Autodesk Inventor part; units mm, degrees
ref_plane "YZ Plane" through (0, 0, 0) normal (1, 0, 0) x (0, 1, 0)
ref_plane "XZ Plane" through (0, 0, 0) normal (0, 1, 0) x (-1, 0, 0)
ref_plane "XY Plane" through (0, 0, 0) normal (0, 0, 1) x (1, 0, 0)
sketch "スケッチ1" plane through (0, 0, 0) normal (0, 0, 1) x (1, 0, 0)
  line L0 (-20, -10) -> (20, -10)
  line L1 (20, -10) -> (20, 10)
  line L2 (20, 10) -> (-20, 10)
  line L3 (-20, 10) -> (-20, -10)
  line L4 (-20, -10) -> (20, 10) construction
  line L5 (20, -10) -> (-20, 10) construction
  line L6 (-18.4, 8.4) -> (18.4, 8.4)
  line L7 (18.4, 8.4) -> (18.4, -8.4)
  line L8 (18.4, -8.4) -> (-18.4, -8.4)
  line L9 (-18.4, -8.4) -> (-18.4, 8.4)
  point P0 (0, 0)
  dimension "d0" = 40
  dimension "d1" = 20
  dimension "d2" = 1.6
extrude "押し出し1" add sketch "スケッチ1" along normal blind 50
chamfer "面取り1" distance 20 angle 45 1 edges at (0, -10, 0)
sketch "スケッチ2" plane through (-20, -10, 50) normal (0, -1, 0) x (1, 0, 0)
  line L0 (0, 0) -> (40, 0)
  line L1 (40, -30) -> (40, 0)
  point P0 (20, -50)
  point P1 (20, -15)
  dimension "d9" = 15
  dimension "d10" = 20
hole "穴1" at (0, -10, 35) direction (0, 1, 0) diameter 15 end through all
properties part number "Pipe4"
Design review of the part built by this model. Coordinates are the model's own, in mm. A direction names the side the tool comes from. Coordinates: 2 decimals unless noted, no trailing zeros. Order: outer loops, then holes, each group sorted by start corner. A loop starts at its lowest first (then second) coordinate and runs counter-clockwise, first axis right, second up.
1) Take a section at D-D, the plane x = 0. Give the boundary of the cut face in (y, z).
2) Take a section at A-A, the plane y = 3.75. Give the boundary of the cut face in (x, z).
3) Take a section at C-C, the plane z = 19. Give the boundary of the cut face in (x, y).
4) Mouldability with a two-part tool opening along Z and no side actions: class faces 3 (the flat face through (-2, -9, 50)), 4 (the flat face through (0, 10, 25)), 5 (the cylindrical face through (-0.33, -9.189, 42.493)) as +Z half, -Z half, draft (parallel to the pull), parting line (faces both ways), or undercut.
5) Take a section at B-B, the plane x = 13. Give the boundary of the cut face in (y, z), and give its area (3 significant figures).
6) Clearance check with flat-ended pins moving along their axes: pin 1 (3 mm diameter, centred on x = -2.5, z = 18, fed in from -Y); pin 2 (5 mm diameter, centred on x = -8.5, z = 16, fed in from -Y). State where each tip first meets the part, or that it passes through.
7) Wall thickness on line 1 along Y through (x, z) = (-15, 26); line 2 along X through (y, z) = (4.5, 36.5); line 3 along X through (y, z) = (9.2, 35): over which ranges is each line inside the solid? List them lowest first.
8) For faces 1 (the flat face through (-2, -9, 19)), 2 (the flat face through (0, 8.4, 25)), list the 3-axis set-ups (+Z, -Z, +X, -X, +Y, -Y) from which the entire face can be reached by the end or side of a thin tool; tool diameter is ignored.
Returned:
1. outline: (-10, 20) - (-8.4, 18.4) - (-8.4, 27.5) - (-10, 27.5) - close; (-10, 42.5) - (-8.4, 42.5) - (-8.4, 50) - (-10, 50) - close; (8.4, 1.6) - (10, 0) - (10, 27.5) - (8.4, 27.5) - close; (8.4, 42.5) - (10, 42.5) - (10, 50) - (8.4, 50) - close
2. outline: (-20, 6.25) - (-18.4, 6.25) - (-18.4, 50) - (-20, 50) - close; (18.4, 6.25) - (20, 6.25) - (20, 50) - (18.4, 50) - close
3. outline: (-20, -9) - (20, -9) - (20, 10) - (-20, 10) - close; hole (-18.4, -8.4) - (18.4, -8.4) - (18.4, 8.4) - (-18.4, 8.4) - close
4. face 3: +Z half
4. face 4: draft
4. face 5: undercut
5. outline: (-10, 20) - (-8.4, 18.4) - (-8.4, 50) - (-10, 50) - close; (8.4, 1.6) - (10, 0) - (10, 50) - (8.4, 50) - close
5. area: 128 mm2
6. pin 1: stops at y = -9.5
6. pin 2: stops at y = -8.5
7. line 1: y = -10 to -8.4, 8.4 to 10
7. line 2: x = -20 to -18.4, 18.4 to 20
7. line 3: x = -20 to -7.5, 7.5 to 20
8. face 1: -Z, +X, -X, -Y
8. face 2: +Z, -Z
